```python
from build123d import *

# Parameters (mm, degrees)
BOSS_EXTRUDE1_DEPTH     = 35
BOSS_EXTRUDE2_START     = -5
BOSS_EXTRUDE2_DEPTH     = 5
BOSS_EXTRUDE3_START     = -5
BOSS_EXTRUDE3_DEPTH     = 5
CUT_EXTRUDE1_DEPTH      = 31.1
SKETCH10_W              = 5
SKETCH10_H              = 3.78
BOSS_EXTRUDE6_DEPTH     = 5
CUT_EXTRUDE4_START      = -10
CUT_EXTRUDE4_DEPTH      = 20
SKETCH12_R              = 1
CUT_EXTRUDE5_DEPTH      = 10
CUT_EXTRUDE11_DEPTH     = 2
SKETCH14_R              = 2.5
CUT_EXTRUDE12_DEPTH     = 2
BOSS_EXTRUDE7_START     = -2
SKETCH15_R              = 2
BOSS_EXTRUDE7_DEPTH     = 5
BOSS_EXTRUDE8_DEPTH     = 6
SKETCH18_W              = 32.6
SKETCH18_H              = 12
BOSS_EXTRUDE9_DEPTH     = 2
SKETCH19_W              = 32.6
SKETCH19_H              = 12
BOSS_EXTRUDE10_DEPTH    = 2
CUT_EXTRUDE13_DEPTH     = 64.083608013
BOSS_EXTRUDE12_START    = -5
BOSS_EXTRUDE12_DEPTH    = 5
SKETCH22_W              = 16
SKETCH22_H              = 32.6
CUT_EXTRUDE14_DEPTH     = 5
SKETCH23_R              = 2
CUT_EXTRUDE15_DEPTH     = 5
SKETCH24_W              = 23.178287832
SKETCH24_H              = 10
CUT_EXTRUDE_THIN1_DEPTH = 5
CUT_EXTRUDE16_DEPTH     = 5
SKETCH26_W              = 16
SKETCH26_H              = 7
BOSS_EXTRUDE13_DEPTH    = 2


with BuildPart() as part:
    # Sketch2 → Boss-Extrude1 (new body)
    with BuildSketch(Plane(origin=(0, 0, 0), x_dir=(0, 0, -1), z_dir=(1, 0, 0))):
        with BuildLine():
            Line((-15, 13.54), (-13.54, 13.54))
            ThreePointArc((-13.54, 13.54), (0, 0), (13.54, 13.54))
            Line((13.54, 13.54), (15, 13.54))
            Line((15, 13.54), (15, -1.46))
            Line((15, -1.46), (0, -1.46))
            Line((0, -1.46), (-15, -1.46))
            Line((-15, -1.46), (-15, 13.54))
        make_face()
    extrude(amount=BOSS_EXTRUDE1_DEPTH)

    # Sketch3 → Boss-Extrude2 (add)
    with BuildSketch(Plane(origin=(35, 0, 0), x_dir=(0, 0, -1), z_dir=(1, 0, 0)).offset(BOSS_EXTRUDE2_START)):
        with BuildLine():
            Line((-13.54, 13.54), (-5, 13.54))
            ThreePointArc((-5, 13.54), (0, 8.54), (5, 13.54))
            Line((5, 13.54), (13.54, 13.54))
            ThreePointArc((13.54, 13.54), (0, 0), (-13.54, 13.54))
        make_face()
    extrude(amount=BOSS_EXTRUDE2_DEPTH)

    # Sketch4 → Boss-Extrude3 (add)
    with BuildSketch(Plane.ZY.offset(BOSS_EXTRUDE3_START)):
        with BuildLine():
            Line((-13.54, 13.54), (-11.78, 13.54))
            ThreePointArc((-11.78, 13.54), (0, 1.76), (11.78, 13.54))
            Line((11.78, 13.54), (13.54, 13.54))
            ThreePointArc((13.54, 13.54), (0, 0), (-13.54, 13.54))
        make_face()
    extrude(amount=-BOSS_EXTRUDE3_DEPTH)

    # Sketch7 → Cut-Extrude1 (cut)
    with BuildSketch(Plane(origin=(0, 0, -15), x_dir=(-1, 0, 0), z_dir=(0, 0, -1))):
        with BuildLine():
            Line((-33.5, -1.74), (-39.5, -1.74))
            Line((-39.5, -1.74), (-39.5, 4.26))
            ThreePointArc((-39.5, 4.26), (-35.257359313, 2.502640687), (-33.5, -1.74))
        make_face()
    extrude(amount=-CUT_EXTRUDE1_DEPTH, mode=Mode.SUBTRACT)

    # Sketch10 → Boss-Extrude6 (add)
    with BuildSketch(Plane(origin=(0, 13.54, 0), x_dir=(1, 0, 0), z_dir=(0, 1, 0))):
        with Locations((7.5, -16.89)):
            Rectangle(SKETCH10_W, SKETCH10_H)
        with Locations((7.5, 16.89)):
            Rectangle(SKETCH10_W, SKETCH10_H)
    extrude(amount=-BOSS_EXTRUDE6_DEPTH)

    # Sketch11 → Cut-Extrude4 (cut)
    with BuildSketch(Plane.ZY.offset(CUT_EXTRUDE4_START)):
        with BuildLine():
            ThreePointArc((15, 13.54), (10.606601722, 2.933398287), (1.2e-08, -1.46))
            Line((1.2e-08, -1.46), (15, -1.46))
            Line((15, -1.46), (15, 13.54))
        make_face()
        with BuildLine():
            ThreePointArc((1.2e-08, -1.46), (-10.606601713, 2.933398278), (-15, 13.54))
            Line((-15, 13.54), (-15, -1.46))
            Line((-15, -1.46), (1.2e-08, -1.46))
        make_face()
    extrude(amount=-CUT_EXTRUDE4_DEPTH, mode=Mode.SUBTRACT)

    # Sketch12 → Cut-Extrude5 (cut)
    with BuildSketch(Plane(origin=(0, 13.54, 0), x_dir=(1, 0, 0), z_dir=(0, 1, 0))):
        with Locations(Location((7.5, -16.04, 0), (0, 0, 270))):
            Circle(SKETCH12_R)
        with Locations(Location((7.5, 16.04, 0), (0, 0, 270))):
            Circle(SKETCH12_R)
        with Locations(Location((32.5, -9.5, 0), (0, 0, 270))):
            Circle(SKETCH12_R)
        with Locations(Location((32.5, 9.5, 0), (0, 0, 270))):
            Circle(SKETCH12_R)
    extrude(amount=-CUT_EXTRUDE5_DEPTH, mode=Mode.SUBTRACT)

    # Sketch13 → Cut-Extrude11 (cut)
    with BuildSketch(Plane(origin=(0, 8.54, 0), x_dir=(1, 0, 0), z_dir=(0, 1, 0))):
        with BuildLine():
            Line((32.5, 12), (35, 12))
            Line((35, 12), (35.753860742, 12))
            Line((35.753860742, 12), (35.753860742, 7))
            Line((35.753860742, 7), (35, 7))
            Line((35, 7), (32.5, 7))
            ThreePointArc((32.5, 7), (31, 7.5), (30.1, 8.8))
            Line((30.1, 8.8), (30.1, 9.5))
            Line((30.1, 9.5), (30.1, 10.2))
            ThreePointArc((30.1, 10.2), (31, 11.5), (32.5, 12))
        make_face()
        with BuildLine():
            Line((32.5, -7), (35, -7))
            Line((35, -7), (35.753860742, -7))
            Line((35.753860742, -7), (35.753860742, -12))
            Line((35.753860742, -12), (32.5, -12))
            ThreePointArc((32.5, -12), (31, -11.5), (30.1, -10.2))
            Line((30.1, -10.2), (30.1, -9.5))
            Line((30.1, -9.5), (30.1, -8.8))
            ThreePointArc((30.1, -8.8), (31, -7.5), (32.5, -7))
        make_face()
    extrude(amount=-CUT_EXTRUDE11_DEPTH, mode=Mode.SUBTRACT)

    # Sketch14 → Cut-Extrude12 (cut)
    with BuildSketch(Plane.XZ.offset(-8.54)):
        with Locations((7.5, 16.04)):
            Circle(SKETCH14_R)
        with Locations((7.5, -16.04)):
            Circle(SKETCH14_R)
    extrude(amount=CUT_EXTRUDE12_DEPTH, mode=Mode.SUBTRACT)

    # Sketch20 → Cut-Extrude13 (cut, through all)
    with BuildSketch(Plane(origin=(35, 0, 0), x_dir=(0, 0, -1), z_dir=(1, 0, 0))):
        with BuildLine():
            Line((15, 8.54), (12.582988516, 8.54))
            ThreePointArc((12.582988516, 8.54), (0.000990149, 0.000672008), (-12.581008218, 8.54))
            Line((-12.581008218, 8.54), (-15, 8.54))
            Line((-15, 8.54), (-15, -1.46))
            Line((-15, -1.46), (15, -1.46))
            Line((15, -1.46), (15, 8.54))
        make_face()
    extrude(amount=-CUT_EXTRUDE13_DEPTH, mode=Mode.SUBTRACT)



with BuildPart() as body_2:
    # Sketch15 → Boss-Extrude7 (new body)
    with BuildSketch(Plane(origin=(0, 0, 0), x_dir=(-1, 0, 0), z_dir=(0, 0, -1)).offset(BOSS_EXTRUDE7_START)):
        with Locations((-47.000109969, 13.54)):
            Circle(SKETCH15_R)
    extrude(amount=-BOSS_EXTRUDE7_DEPTH)

    # Sketch23 → Cut-Extrude15 (cut)
    with BuildSketch(Plane(origin=(0, 0, 2), x_dir=(-1, 0, 0), z_dir=(0, 0, -1))):
        with Locations((-47.000109969, 13.54)):
            Circle(SKETCH23_R)
    extrude(amount=-CUT_EXTRUDE15_DEPTH, mode=Mode.SUBTRACT)


with BuildPart() as body_3:
    # Sketch16 → Boss-Extrude8 (new, symmetric)
    with BuildSketch(Plane(origin=(47, 0, 0), x_dir=(0, 0, -1), z_dir=(1, 0, 0))):
        Polygon((-18, 11.94), (-18, 8.54), (-49.1, 8.54), (-49.1, 6.54), (-16.5, 6.54), (-16.5, 11.94), align=None)
    extrude(amount=BOSS_EXTRUDE8_DEPTH, both=True)

    # Sketch18 → Boss-Extrude9 (add)
    with BuildSketch(Plane.ZY.offset(-41)):
        with Locations((32.8, 12.54)):
            Rectangle(SKETCH18_W, SKETCH18_H)
    extrude(amount=BOSS_EXTRUDE9_DEPTH)

    # Sketch19 → Boss-Extrude10 (add)
    with BuildSketch(Plane(origin=(53, 0, 0), x_dir=(0, 0, -1), z_dir=(1, 0, 0))):
        with Locations((-32.8, 12.54)):
            Rectangle(SKETCH19_W, SKETCH19_H)
    extrude(amount=BOSS_EXTRUDE10_DEPTH)


with BuildPart() as part_1:
    add(part.part)

    add(body_3.part)  # Boss-Extrude12 merges body 3
    # Sketch21 → Boss-Extrude12 (add)
    with BuildSketch(Plane(origin=(0, 13.54, 0), x_dir=(1, 0, 0), z_dir=(0, 1, 0)).offset(BOSS_EXTRUDE12_START)):
        Polygon((35, -15), (39, -19), (39, -24), (30, -15), align=None)
        Polygon((25, -15), (39, -29), (39, -34), (20, -15), (19.142135624, -14.142135624), (24.142135624, -14.142135624), align=None)
    extrude(amount=BOSS_EXTRUDE12_DEPTH)

    # Sketch22 → Cut-Extrude14 (cut)
    with BuildSketch(Plane(origin=(0, 13.54, 0), x_dir=(1, 0, 0), z_dir=(0, 1, 0))):
        with Locations((47, -32.8)):
            Rectangle(SKETCH22_W, SKETCH22_H)
    extrude(amount=CUT_EXTRUDE14_DEPTH, mode=Mode.SUBTRACT)

    # Sketch24 → Cut-Extrude-Thin1 (cut)
    with BuildSketch(Plane(origin=(35, 0, 0), x_dir=(0, 0, -1), z_dir=(1, 0, 0))):
        with Locations((0.000990149, 1.54)):
            Rectangle(SKETCH24_W, SKETCH24_H)
        with BuildLine():
            ThreePointArc((-11.587661518, 6.54), (0, 0.002130911), (11.587661518, 6.54))
            Line((11.587661518, 6.54), (20.14710425, 1.369319183))
            ThreePointArc((20.14710425, 1.369319183), (0, -9.997869089), (-20.14710425, 1.369319183))
            Line((-20.14710425, 1.369319183), (-11.587661518, 6.54))
        make_face()
    extrude(amount=-CUT_EXTRUDE_THIN1_DEPTH, mode=Mode.SUBTRACT)

    # Sketch25 → Cut-Extrude16 (cut)
    with BuildSketch(Plane.XY.offset(18)):
        with BuildLine():
            Line((45.047915657, 11.94), (48.952084343, 11.94))
            ThreePointArc((48.952084343, 11.94), (47, 11.083618243), (45.047915657, 11.94))
        make_face()
    extrude(amount=-CUT_EXTRUDE16_DEPTH, mode=Mode.SUBTRACT)

    # Sketch26 → Boss-Extrude13 (add)
    with BuildSketch(Plane.XY.offset(49.1)):
        with Locations((47, 10.04)):
            Rectangle(SKETCH26_W, SKETCH26_H)
    extrude(amount=BOSS_EXTRUDE13_DEPTH)


solid = part_1.part
```
Design review of the part built by this model. Coordinates are the model's own, in mm. A direction names the side the tool comes from. Give positions to 0.01 mm unless a question says otherwise; leave off trailing zeros. Order: outer loops, then holes, each group sorted by start corner. A loop starts at its lowest first (then second) coordinate and runs counter-clockwise, first axis right, second up. Notation, with made-up numbers: (27.5, -24.75) -> (58.5, -24.75) arc R19 cw to (58.5, -5.75) -> close; hole circle Ø9 at (70, 38.5). An arc over 180 degrees is marked (long way). Write item = value, one per line. Start each with the question number.
(1) We need section C-C on x = 7.5. Write out the cut boundary in (y, z), plus the area to 3 significant figures.
(2) For pin 1 (5 mm diameter, centred on y = 1.5, z = 0, fed in from -X); pin 2 (4 mm diameter, centred on y = 9, z = -2.5, fed in from -X); pin 3 (4 mm diameter, centred on x = 33, z = -0.5, fed in from -Y); pin 4 (3 mm diameter, centred on x = 44.5, y = 3.5, fed in from -Z), all flat-tipped, find the tip position at first contact; note any pin that passes through.
(3) To check wall thickness, follow line 1 along X through (y, z) = (12.2, 9.5); line 2 along X through (y, z) = (9.75, 48.5); line 3 along X through (y, z) = (10.3, 16.04). State the ranges of each line that lie inside material, in increasing order.
(4) Mouldability with a two-part tool opening along X and no side actions: class faces 1 (the face through (55, 10, 34)), 2 (the face through (34, 8.54, 9)), 3 (the face through (7.54, 11.08, -17.04)) as +X half, -X half, draft (parallel to the pull), parting line (faces both ways), or undercut.
(5) For faces 4 (the face through (31, 7.6, 7.5)), 5 (the face through (35, 8, 0)), 6 (the face through (47, 10, 18)), list the 3-axis set-ups (+Z, -Z, +X, -X, +Y, -Y) from which the entire face can be reached by the end or side of a thin tool; tool diameter is ignored.
(6) We need section A-A on x = 15.5. Write out the cut boundary in (y, z), plus the area to 3 significant figures.
(7) We need section B-B on z = 26. Write out the cut boundary in (x, y).
(8) We need section D-D on y = 4.75. Write out the cut boundary in (x, z).
Numbers:
q1.outline = (8.54, -18.78) -> (13.54, -18.78) -> (13.54, -17.04) -> (8.54, -17.04) -> close; (8.54, -15.04) -> (13.54, -15.04) -> (13.54, -11.78) arc R11.78 cw to (13.54, 11.78) -> (13.54, 15.04) -> (8.54, 15.04) -> (8.54, 12.58) arc R13.54 ccw to (8.54, -12.58) -> close; (8.54, 17.04) -> (13.54, 17.04) -> (13.54, 18.78) -> (8.54, 18.78) -> close
q1.area = 106 mm^2
q2.pin_1 = 5
q2.pin_2 = 30
q2.pin_3 = 6.54
q2.pin_4 = through
q3.line_1 = 30 to 31.5, 33.5 to 35
q3.line_2 = 39 to 41, 53 to 55
q3.line_3 = 5 to 6.5, 8.5 to 10, 21.04 to 26.04, 31.04 to 36.04
q4.face_1 = +X half
q4.face_2 = draft
q4.face_3 = undercut
q5.face_4 = +X, -Y
q5.face_5 = -Z, +X, +Y, -Y
q5.face_6 = +Y
q6.outline = (8.54, -14.14) arc R15 ccw to (13.54, -15) -> (13.54, -13.54) arc R13.54 cw to (8.54, -12.58) -> close; (8.54, 12.58) arc R13.54 cw to (13.54, 13.54) -> (13.54, 15) arc R15 ccw to (8.54, 14.14) -> close
q6.area = 14.9 mm^2
q7.outline = (31, 8.54) -> (36, 8.54) -> (36, 13.54) -> (31, 13.54) -> close; (39, 6.54) -> (55, 6.54) -> (55, 13.54) -> (53, 13.54) -> (53, 8.54) -> (41, 8.54) -> (41, 13.54) -> (39, 13.54) -> close
q8.outline = (5, -10.3) -> (10, -10.3) -> (10, -7.84) -> (5, -7.84) -> close; (5, 7.84) -> (10, 7.84) -> (10, 10.3) -> (5, 10.3) -> close
